The listing builds one solid part. Answer for the finished solid, in the listing's coordinates (mm). Round coordinates to 2 decimals unless told otherwise and drop trailing zeros. Write each loop counter-clockwise with the first axis right and the second up, starting at its lowest first coordinate (ties: lowest second). Pieces come first, ordered by that corner, then holes.
(1) A cutting plane is placed at A-A, the plane x = 0. Give the vertices of the cut face in (y, z), and give its area (3 significant figures).
(2) Find the intervals of material crossed by probe 1 along Z at (x, y) = (0.5, 2.75); probe 2 along Z at (x, y) = (0, 1), in increasing order.
(3) The mould has two halves that part along Z. Classify faces 1 (the face through (0, 0, 0)), 2 (the face through (0, -4.762, 100)), 3 (the face through (0.732, -0.067, 12.823)), 4 (the face through (0, 0, 203.2)): +Z half, -Z half, draft (parallel to the pull), parting line (faces both ways), or undercut.
(4) This flat-tipped pin is pushed along its axis until it touches: pin 1 Ø4 at (x, z) = (0, 9.525) entering from +Y. Where does it stop, or does it pass through?
from build123d import *

# Parameters (mm, degrees)
SKETCH1_W               = 19.05
SKETCH1_H               = 9.525
BOSS_EXTRUDE1_DEPTH     = 203.2
F_1_4_CLEARANCE_HOLE1_D = 6.7564


with BuildPart() as part:
    # Sketch1 → Boss-Extrude1 (new body)
    with BuildSketch(Plane.XY):
        Rectangle(SKETCH1_W, SKETCH1_H)
    extrude(amount=BOSS_EXTRUDE1_DEPTH)

    # 1/4 Clearance Hole1 (through all)
    with Locations(Plane(origin=(0, 4.7625, 0), x_dir=(1, 0, 0), z_dir=(0, 1, 0))):
        with Locations((0, -9.525)):
            Hole(F_1_4_CLEARANCE_HOLE1_D / 2)


solid = part.part
Solutions:
1. outline: (-4.76, 0) - (4.76, 0) - (4.76, 6.15) - (-4.76, 6.15) - close; (-4.76, 12.9) - (4.76, 12.9) - (4.76, 203.2) - (-4.76, 203.2) - close
1. area: 1,870 mm2
2. probe 1: z = 0 to 6.18, 12.87 to 203.2
2. probe 2: z = 0 to 6.15, 12.9 to 203.2
3. face 1: -Z half
3. face 2: draft
3. face 3: undercut
3. face 4: +Z half
4. pin 1: passes through
